```python
from build123d import *

# Parameters (mm, degrees)
SKETCH1_W           = 10
SKETCH1_H           = 10
BOSS_EXTRUDE1_DEPTH = 20
SKETCH2_W           = 20
SKETCH2_H           = 20
CUT_EXTRUDE1_DEPTH  = 10
BOSS_EXTRUDE2_DEPTH = 10
CUT_EXTRUDE2_DEPTH  = 25
SKETCH5_W           = 12.5
SKETCH5_H           = 7.5
CUT_EXTRUDE3_DEPTH  = 25
FILLET6_R           = 3
FILLET7_R           = 2.5
FILLET8_R           = 2.5
FILLET9_R           = 2.5
FILLET10_R          = 2.5


# Some blends are built 0.0001 mm under size
with BuildPart() as part:
    # Sketch1 → Boss-Extrude1 (new body)
    with BuildSketch(Plane(origin=(0, 0, 0), x_dir=(1, 0, 0), z_dir=(0, 1, 0))):
        Polygon((0, 10), (-10, 10), (-10, -10), (10, -10), (10, 0), (0, 0), align=None)
        with Locations((5, 5)):
            Rectangle(SKETCH1_W, SKETCH1_H)
    extrude(amount=BOSS_EXTRUDE1_DEPTH)

    # Sketch2 → Cut-Extrude1 (cut)
    with BuildSketch(Plane(origin=(0, 20, 0), x_dir=(1, 0, 0), z_dir=(0, 1, 0))):
        with Locations((10, 10)):
            Rectangle(SKETCH2_W, SKETCH2_H)
    extrude(amount=-CUT_EXTRUDE1_DEPTH, mode=Mode.SUBTRACT)

    # Sketch3 → Boss-Extrude2 (add)
    with BuildSketch(Plane(origin=(0, 0, 0), x_dir=(-1, 0, 0), z_dir=(0, 0, -1))):
        with BuildLine():
            Line((-1.464466094, 13.535533906), (-3.535533906, 11.464466094))
            ThreePointArc((-3.535533906, 11.464466094), (-5.15765065, 10.380602337), (-7.071067812, 10))
            Line((-7.071067812, 10), (0, 10))
            Line((0, 10), (0, 17.071067812))
            ThreePointArc((0, 17.071067812), (-0.380602337, 15.15765065), (-1.464466094, 13.535533906))
        make_face()
    extrude(amount=BOSS_EXTRUDE2_DEPTH)

    # Sketch4 → Cut-Extrude2 (cut)
    with BuildSketch(Plane(origin=(0, 20, 0), x_dir=(1, 0, 0), z_dir=(0, 1, 0))):
        Polygon((-2.5, -2.5), (-2.5, 10), (-10, 10), (-10, -10), (10, -10), (10, -2.5), align=None)
    extrude(amount=-CUT_EXTRUDE2_DEPTH, mode=Mode.SUBTRACT)

    # Sketch5 → Cut-Extrude3 (cut)
    with BuildSketch(Plane(origin=(10, 0, 0), x_dir=(0, 0, -1), z_dir=(1, 0, 0))):
        with Locations((3.75, 3.75)):
            Rectangle(SKETCH5_W, SKETCH5_H)
    extrude(amount=-CUT_EXTRUDE3_DEPTH, mode=Mode.SUBTRACT)

    # Fillet6
    fillet6_edges = [part.edges().sort_by_distance(p)[0] for p in [
        (-2.5, 13.75, 2.5),
    ]]
    fillet(fillet6_edges, radius=FILLET6_R)

    # Fillet7
    # the kernel refuses this fillet: 2.5 mm, written as the material it takes off along each edge
    with BuildSketch(Plane(origin=(16.25, 20, 2.5), x_dir=(0, 0, -1), z_dir=(-1, 0, 0)), Plane(origin=(-2.5, 20, -0.5), x_dir=(1, 0, 0), z_dir=(0, 0, -1))) as fillet7_piece_1:
        with BuildLine():
            CenterArc((FILLET7_R, FILLET7_R), FILLET7_R, 180, 90)
            Line((0, FILLET7_R), (0, 0))
            Line((0, 0), (FILLET7_R, 0))
        make_face()
    extrude(amount=15.75, mode=Mode.SUBTRACT)
    with BuildSketch(Plane(origin=(0.5, 20, -0.5), x_dir=(-1, 0, 0), z_dir=(0, 0, -1))) as fillet7_piece_2:
        with BuildLine():
            CenterArc((3 - FILLET7_R, -FILLET7_R), FILLET7_R, 0, 90)
            Line((3, -FILLET7_R), (3, 0))
            Line((3, 0), (3 - FILLET7_R, 0))
        make_face()
    revolve(axis=Axis((0.5, 20, -0.5), (0, 1, 0)), revolution_arc=90, mode=Mode.SUBTRACT)

    # Fillet8
    fillet8_edges = [part.edges().sort_by_distance(p)[0] for p in [
        (-2.5, 7.5, -5.25),
        (5.25, 7.5, 2.5),
        (-1.621320344, 7.5, 1.621320344),
    ]]
    fillet(fillet8_edges, radius=FILLET8_R)

    # Fillet9
    fillet9_edges = [part.edges().sort_by_distance(p)[0] for p in [
        (5, 7.5, -10),
        (-1.767766953, 19.267766953, -10),
        (-2.5, 13.75, -10),
        (10, 19.267766953, 1.767766953),
        (10, 13.75, 2.5),
        (10, 7.5, -5),
        (-1.767766953, 8.232233047, -10),
        (10, 8.232233047, 1.767766953),
    ]]
    fillet(fillet9_edges, radius=FILLET9_R - 0.0001)  # a hair under: the kernel refuses the full size

    # Fillet10
    # the kernel refuses this fillet: 2.5 mm, written as the material it takes off along each edge
    with BuildSketch(Plane(origin=(7.5, 7.5, -7.5), x_dir=(0, 0, -1), z_dir=(-1, 0, 0))) as fillet10_piece_1:
        with BuildLine():
            CenterArc((0.0001, -2.4999), 2.4999, 0, 90)
            Line((2.5, -2.4999), (2.5, 0))
            Line((2.5, 0), (0.0001, 0))
        make_face()
    revolve(axis=Axis((7.5, 7.5, -7.5), (0, -1, 0)), revolution_arc=90, mode=Mode.SUBTRACT)
    with BuildSketch(Plane(origin=(10, 7.5, -10), x_dir=(-1, 0, 0), z_dir=(0, 1, 0))) as fillet10_piece_2:
        with BuildLine():
            CenterArc((FILLET10_R, FILLET10_R), FILLET10_R, 180, 90)
            Line((0, FILLET10_R), (0, 0))
            Line((0, 0), (FILLET10_R, 0))
        make_face()
    extrude(amount=8.75, mode=Mode.SUBTRACT)


solid = part.part
```
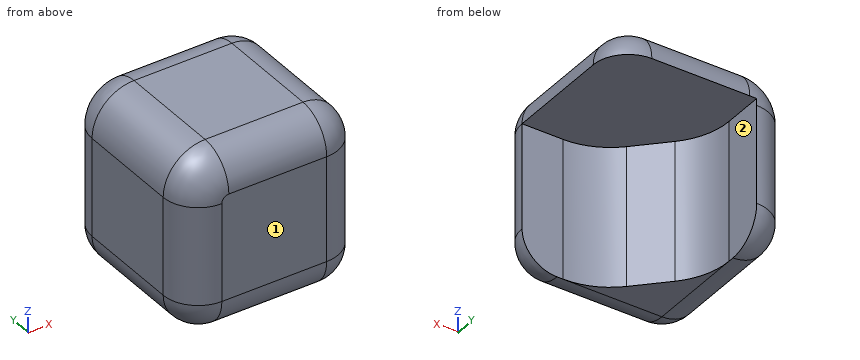
Here's how the part is built. I have some questions about the finished solid (model axes, mm). Face numbers are marked on the shaded views. A direction names the side the tool comes from. Round coordinates to 2 decimals unless told otherwise and drop trailing zeros. Loops run counter-clockwise (first coordinate to the right, second up) from the corner with the lowest first, then second, coordinate; pieces in that order, holes last.
1. If I drill on probe 1 along Z at (x, y) = (3.5, 12); probe 2 along X at (y, z) = (16.25, -0.5); probe 3 along X at (y, z) = (9.5, -6), over which ranges is the centre line in solid material (lowest first)?
Answers:
probe 1: z = 0 to 2.5
probe 2: x = -2.5 to 0.07
probe 3: x = -2.45 to 9.95
2. For the marked faces 1 and 2, which set-ups out of +Z, -Z, +X, -X, +Y, -Y let a thin tool reach every point of the face, with its end or its side?
Answers:
face 1: +Z, -Z, +X, -X, -Y
face 2: -Z, +X, +Y
3. Will these pins go through, and if not, where does the flat tip stop? pin 1 (3 mm diameter, centred on y = 19, z = -6.5, fed in from +X); pin 2 (4 mm diameter, centred on x = 3.5, y = 15, fed in from -Z); pin 3 (2.5 mm diameter, centred on x = 8.5, z = -6, fed in from +Y).
Answers:
pin 1: stops at x = 0
pin 2: stops at z = 0
pin 3: stops at y = 10
4. Suppose I cut it at D-D, the plane x = 4.25. Please give me the cut outline in (y, z).
Answers:
outline: (7.5, -7.5) arc R2.5 ccw to (10, -10) - (10.87, -10) - (10.87, 0) - (20, 0) arc R2.5 ccw to (17.5, 2.5) - (10, 2.5) arc R2.5 ccw to (7.5, 0) - close
5. Suppose I cut it at C-C, the plane x = 2.25. Please give me the cut outline in (y, z).
Answers:
outline: (7.5, -7.5) arc R2.5 ccw to (10, -10) - (12.75, -10) - (12.75, 0) - (20, 0) arc R2.5 ccw to (17.5, 2.5) - (10, 2.5) arc R2.5 ccw to (7.5, 0) - close
